Geometry check sheet. Reference: the model listing, model coordinates, mm. A direction names the side the tool comes from. Give positions to 0.01 mm unless a question says otherwise; leave off trailing zeros. Loops run counter-clockwise (first coordinate to the right, second up) from the corner with the lowest first, then second, coordinate; pieces in that order, holes last. Notation, with made-up numbers: (35, -8.75) -> (55, -8.75) arc R8 cw to (55, -2.75) -> close; hole circle Ø4 at (68.25, 26.5). An arc over 180 degrees is marked (long way). One line per item, written item: value. Start each with the question number.
(1) Draft check along X on faces 1 (the face through (73.908, 20.226, 1.972)), 2 (the face through (106.925, -39, 14)), 3 (the face through (106, -9, 29.4)). Enter one of: pulls with the +X half, pulls with the -X half, needs draft (parallel to the pull), parting line crosses it, or undercut.
(2) Sectioned sample at D-D, the plane z = 24.25. Record the cut outline in (x, y) (3 decimals).
(3) Sectioned sample at A-A, the plane x = 65. Record the cut outline in (y, z) (3 decimals), then the cut area to 3 significant figures.
(4) Sectioned sample at C-C, the plane y = -17. Record the cut outline in (x, z) (3 decimals).
(5) Sectioned sample at B-B, the plane z = 19.05. Record the cut outline in (x, y) (3 decimals), then the cut area to 3 significant figures.
(6) Tool access check on faces 4 (the face through (106.02, -38.669, 0.955)), 5 (the face through (2, 4, 6)), 6 (the face through (4, 13, 5)), 7 (the face through (2, 23.25, 6)). Record the directions out of +Z, -Z, +X, -X, +Y, -Y that give a thin tool (end or side, any length) a straight path to the whole face; none if there is none.
(7) Gauge pin test, flat ends, axial feed: pin 1 Ø3 at (x, y) = (25.5, 11.5) entering from -Z; pin 2 Ø12.5 at (y, z) = (-5.5, 20) entering from -X (3 decimals); pin 3 Ø6.5 at (x, y) = (65, 13.625) entering from +Z; pin 4 Ø4 at (y, z) = (-21.5, 18.5) entering from +X (3 decimals). Record the tip position at first contact, or that the pin passes through.
(8) Scan lines: line 1 along Y through (x, z) = (72, 0.9) (3 decimals); line 2 along Y through (x, z) = (105.1, 19.05) (3 decimals); line 3 along Y through (x, z) = (71.5, 3.25). Record each from-to range of solid material in increasing order. Write a range as from..to.
from build123d import *

# Parameters (mm, degrees)
SKETCH1_R                      = 2
PROFILEBOSS_EXTRUDE1_DEPTH     = 4
CORNERBOSS_EXTRUDE2_DEPTH      = 0.0001
CORNERBOSS_EXTRUDE2_DEPTH_BACK = 25.4
SKETCH2_W                      = 4
SKETCH2_H                      = 91.675
BOSS_EXTRUDE3_DEPTH            = 0.0001
BOSS_EXTRUDE3_DEPTH_BACK       = 2.6
SKETCH3_W                      = 4
SKETCH3_H                      = 19.25
BOSS_EXTRUDE4_DEPTH            = 0.0001
BOSS_EXTRUDE4_DEPTH_BACK       = 2
SKETCH5_W                      = 8
SKETCH5_H                      = 19.25
FILLET1_R                      = 2
CHAMFER1_SIZE                  = 4
VSMOUNTHOLECUT_EXTRUDE1_REACH  = 126.934
SKETCH6_R                      = 3
SKETCH7_W                      = 29.4
SKETCH7_H                      = 40.875
THICKSIDEBOSS_EXTRUDE5_DEPTH   = 3.175
FILLET3_R                      = 3.175


with BuildPart() as part:
    # Sketch1 → ProfileBoss-Extrude1 (new body)
    with BuildSketch(Plane.XY):
        Polygon((0, 0), (81.525, 0), (81.525, -64.425), (106.925, -64.425), (106.925, 27.25), (0, 27.25), align=None)
        with Locations((72, 19.625)):
            Circle(SKETCH1_R, mode=Mode.SUBTRACT)
        with Locations((72, 7.625)):
            Circle(SKETCH1_R, mode=Mode.SUBTRACT)
        with Locations((65, 13.625)):
            Circle(SKETCH1_R, mode=Mode.SUBTRACT)
    extrude(amount=PROFILEBOSS_EXTRUDE1_DEPTH)

    # Sketch2 → CornerBoss-Extrude2 (add, two sides: drawn at the far end of the back side and taken through both)
    with BuildSketch(Plane(origin=(0, 0, 4), x_dir=(-1, 0, 0), z_dir=(0, 0, -1)).offset(-CORNERBOSS_EXTRUDE2_DEPTH_BACK)):
        with Locations((-104.925, -18.5875)):
            Rectangle(SKETCH2_W, SKETCH2_H)
    extrude(amount=CORNERBOSS_EXTRUDE2_DEPTH + CORNERBOSS_EXTRUDE2_DEPTH_BACK)

    # Sketch3 → Boss-Extrude3 (add, two sides: drawn at the far end of the back side and taken through both)
    with BuildSketch(Plane(origin=(0, 0, 4), x_dir=(-1, 0, 0), z_dir=(0, 0, -1)).offset(-BOSS_EXTRUDE3_DEPTH_BACK)):
        with Locations((-2, 13.625)):
            Rectangle(SKETCH3_W, SKETCH3_H)
    extrude(amount=BOSS_EXTRUDE3_DEPTH + BOSS_EXTRUDE3_DEPTH_BACK)

    # Sketch5 → Boss-Extrude4 (add, two sides: drawn at the far end of the back side and taken through both)
    with BuildSketch(Plane(origin=(0, 0, 6.6), x_dir=(-1, 0, 0), z_dir=(0, 0, -1)).offset(-BOSS_EXTRUDE4_DEPTH_BACK)):
        with Locations((-4, 13.625)):
            Rectangle(SKETCH5_W, SKETCH5_H)
    extrude(amount=BOSS_EXTRUDE4_DEPTH + BOSS_EXTRUDE4_DEPTH_BACK)

    # Fillet1
    fillet1_edges = [part.edges().sort_by_distance(p)[0] for p in [
        (8, 4, 7.59995),
        (8, 23.25, 7.59995),
    ]]
    fillet(fillet1_edges, radius=FILLET1_R)

    # Chamfer1
    chamfer1_edges = [part.edges().sort_by_distance(p)[0] for p in [
        (0, 27.25, 2),
        (0, 0, 2),
    ]]
    chamfer(chamfer1_edges, length=CHAMFER1_SIZE)

    # Sketch6 → VSMountHoleCut-Extrude1 (cut, up to next)
    with BuildSketch(Plane.ZY.offset(-102.925), mode=Mode.PRIVATE) as vsmountholecut_extrude1_sk1:
        with Locations((19.05, -39.025)):
            Circle(SKETCH6_R)
    vsmountholecut_extrude1_tool1 = extrude(vsmountholecut_extrude1_sk1.sketch, amount=-VSMOUNTHOLECUT_EXTRUDE1_REACH, mode=Mode.PRIVATE) & part.part
    add(vsmountholecut_extrude1_tool1.solids().sort_by_distance((102.925, -39.025, 19.05))[0], mode=Mode.SUBTRACT)

    # Sketch7 → ThickSideBoss-Extrude5 (add)
    with BuildSketch(Plane(origin=(106.925, 0, 0), x_dir=(0, 0, -1), z_dir=(1, 0, 0))):
        with Locations((-14.7, 6.8125)):
            Rectangle(SKETCH7_W, SKETCH7_H)
    extrude(amount=THICKSIDEBOSS_EXTRUDE5_DEPTH)

    # Fillet3
    fillet3_edges = [part.edges().sort_by_distance(p)[0] for p in [
        (106.925, -39.025, 0),
        (110.1, 6.8125, 0),
    ]]
    fillet(fillet3_edges, radius=FILLET3_R - 0.0001)  # a hair under: the kernel refuses the full size


solid = part.part
Calculated:
1. face 1: undercut
1. face 2: pulls with the +X half
1. face 3: needs draft
2. outline: (102.925, -64.425) -> (106.925, -64.425) -> (106.925, -13.625) -> (110.1, -13.625) -> (110.1, 27.25) -> (102.925, 27.25) -> close
3. outline: (0, 0) -> (11.625, 0) -> (11.625, 4) -> (0, 4) -> close; (15.625, 0) -> (27.25, 0) -> (27.25, 4) -> (15.625, 4) -> close
3. area: 93.0 mm2
4. outline: (81.525, 0) -> (103.75, 0) arc R3.175 ccw to (106.925, 3.175) -> (106.925, 29.4) -> (102.925, 29.4) -> (102.925, 4) -> (81.525, 4) -> close
5. outline: (102.925, -64.425) -> (106.925, -64.425) -> (106.925, -42.025) -> (102.925, -42.025) -> close; (102.925, -36.025) -> (106.925, -36.025) -> (106.925, -13.625) -> (110.1, -13.625) -> (110.1, 27.25) -> (102.925, 27.25) -> close
5. area: 472 mm2
6. face 4: -Z, +X, -Y
6. face 5: +Z, -X, -Y
6. face 6: +Y, -Y
6. face 7: +Z, -X, +Y
7. pin 1: stops at z = 0
7. pin 2: stops at x = 102.925
7. pin 3: stops at z = 4
7. pin 4: stops at x = 106.925
8. line 1: y = 0..5.625, 9.625..17.625, 21.625..27.25
8. line 2: y = -64.425..-42.025, -36.025..27.25
8. line 3: y = 0..5.69, 9.56..17.69, 21.56..27.25
